```python
from build123d import *

# Parameters (mm, degrees)
SKETCH1_W               = 166
SKETCH1_H               = 196
SKETCH1_W_2             = 130
SKETCH1_H_2             = 160
BOSS_EXTRUDE1_DEPTH     = 10
CUT_EXTRUDE1_REACH      = 168
SKETCH2_R               = 2.38125
CUT_EXTRUDE2_DEPTH      = 167
SKETCH5_R               = 2.38125
CUT_EXTRUDE4_DEPTH      = 1
CUT_EXTRUDE4_DEPTH_BACK = 197
CUT_EXTRUDE5_REACH      = 12
SKETCH6_R               = 1.75
CUT_EXTRUDE7_REACH      = 22
SKETCH8_W               = 130
SKETCH8_H               = 4.5
CHAMFER9_SIZE           = 7
CHAMFER10_SIZE          = 3
CUT_EXTRUDE8_REACH      = 22
SKETCH9_R               = 1.190625
CHAMFER11_SIZE          = 3


with BuildPart() as part:
    # Sketch1 → Boss-Extrude1 (new body, symmetric)
    with BuildSketch(Plane(origin=(0, 0, 0), x_dir=(1, 0, 0), z_dir=(0, 1, 0))):
        Rectangle(SKETCH1_W, SKETCH1_H)
        Rectangle(SKETCH1_W_2, SKETCH1_H_2, mode=Mode.SUBTRACT)
    extrude(amount=BOSS_EXTRUDE1_DEPTH, both=True)

    # Sketch2 → Cut-Extrude1 (cut, up to next)
    with BuildSketch(Plane(origin=(83, 0, 0), x_dir=(0, 0, -1), z_dir=(1, 0, 0)), mode=Mode.PRIVATE) as cut_extrude1_sk1:
        Circle(SKETCH2_R)
    cut_extrude1_tool1 = extrude(cut_extrude1_sk1.sketch, amount=-CUT_EXTRUDE1_REACH, mode=Mode.PRIVATE) & part.part
    add(cut_extrude1_tool1.solids().sort_by_distance((83, 0, 0))[0], mode=Mode.SUBTRACT)

    # Sketch3 → Cut-Extrude2 (cut, through all)
    with BuildSketch(Plane.ZY.offset(83)):
        with BuildLine():
            ThreePointArc((-2.38125, 0), (0, 2.38125), (2.38125, 0))
            Line((2.38125, 0), (11, 0))
            Line((11, 0), (11, 10))
            Line((11, 10), (-11, 10))
            Line((-11, 10), (-11, 0))
            Line((-11, 0), (-2.38125, 0))
        make_face()
        with BuildLine():
            ThreePointArc((-2.38125, 0), (0, -2.38125), (2.38125, 0))
            Line((2.38125, 0), (-2.38125, 0))
        make_face()
        with BuildLine():
            Line((-2.38125, 0), (2.38125, 0))
            ThreePointArc((2.38125, 0), (0, 2.38125), (-2.38125, 0))
        make_face()
    extrude(amount=-CUT_EXTRUDE2_DEPTH, mode=Mode.SUBTRACT)

    # Sketch5 → Cut-Extrude4 (cut, two sides)
    with BuildSketch(Plane.XY.offset(98)) as cut_extrude4_sk:
        Circle(SKETCH5_R)
    extrude(amount=CUT_EXTRUDE4_DEPTH, mode=Mode.SUBTRACT)
    extrude(cut_extrude4_sk.sketch, amount=-CUT_EXTRUDE4_DEPTH_BACK, mode=Mode.SUBTRACT)

    # Sketch6 → Cut-Extrude5 (cut, up to next)
    with BuildSketch(Plane(origin=(0, 0, 0), x_dir=(1, 0, 0), z_dir=(0, 1, 0)), mode=Mode.PRIVATE) as cut_extrude5_sk1:
        with Locations((-69, 6.8)):
            Circle(SKETCH6_R)
    cut_extrude5_tool1 = extrude(cut_extrude5_sk1.sketch, amount=-CUT_EXTRUDE5_REACH, mode=Mode.PRIVATE) & part.part
    add(cut_extrude5_tool1.solids().sort_by_distance((-69, 0, -6.8))[0], mode=Mode.SUBTRACT)
    # Sketch6 → Cut-Extrude5 (cut, up to next)
    with BuildSketch(Plane(origin=(0, 0, 0), x_dir=(1, 0, 0), z_dir=(0, 1, 0)), mode=Mode.PRIVATE) as cut_extrude5_sk2:
        with Locations((-69, -6.8)):
            Circle(SKETCH6_R)
    cut_extrude5_tool2 = extrude(cut_extrude5_sk2.sketch, amount=-CUT_EXTRUDE5_REACH, mode=Mode.PRIVATE) & part.part
    add(cut_extrude5_tool2.solids().sort_by_distance((-69, 0, 6.8))[0], mode=Mode.SUBTRACT)
    # Sketch6 → Cut-Extrude5 (cut, up to next)
    with BuildSketch(Plane(origin=(0, 0, 0), x_dir=(1, 0, 0), z_dir=(0, 1, 0)), mode=Mode.PRIVATE) as cut_extrude5_sk3:
        with Locations((-79, -6.8)):
            Circle(SKETCH6_R)
    cut_extrude5_tool3 = extrude(cut_extrude5_sk3.sketch, amount=-CUT_EXTRUDE5_REACH, mode=Mode.PRIVATE) & part.part
    add(cut_extrude5_tool3.solids().sort_by_distance((-79, 0, 6.8))[0], mode=Mode.SUBTRACT)
    # Sketch6 → Cut-Extrude5 (cut, up to next)
    with BuildSketch(Plane(origin=(0, 0, 0), x_dir=(1, 0, 0), z_dir=(0, 1, 0)), mode=Mode.PRIVATE) as cut_extrude5_sk4:
        with Locations((-79, 6.8)):
            Circle(SKETCH6_R)
    cut_extrude5_tool4 = extrude(cut_extrude5_sk4.sketch, amount=-CUT_EXTRUDE5_REACH, mode=Mode.PRIVATE) & part.part
    add(cut_extrude5_tool4.solids().sort_by_distance((-79, 0, -6.8))[0], mode=Mode.SUBTRACT)
    # Sketch6 → Cut-Extrude5 (cut, up to next)
    with BuildSketch(Plane(origin=(0, 0, 0), x_dir=(1, 0, 0), z_dir=(0, 1, 0)), mode=Mode.PRIVATE) as cut_extrude5_sk5:
        with Locations((79, 6.8)):
            Circle(SKETCH6_R)
    cut_extrude5_tool5 = extrude(cut_extrude5_sk5.sketch, amount=-CUT_EXTRUDE5_REACH, mode=Mode.PRIVATE) & part.part
    add(cut_extrude5_tool5.solids().sort_by_distance((79, 0, -6.8))[0], mode=Mode.SUBTRACT)
    # Sketch6 → Cut-Extrude5 (cut, up to next)
    with BuildSketch(Plane(origin=(0, 0, 0), x_dir=(1, 0, 0), z_dir=(0, 1, 0)), mode=Mode.PRIVATE) as cut_extrude5_sk6:
        with Locations((79, -6.8)):
            Circle(SKETCH6_R)
    cut_extrude5_tool6 = extrude(cut_extrude5_sk6.sketch, amount=-CUT_EXTRUDE5_REACH, mode=Mode.PRIVATE) & part.part
    add(cut_extrude5_tool6.solids().sort_by_distance((79, 0, 6.8))[0], mode=Mode.SUBTRACT)
    # Sketch6 → Cut-Extrude5 (cut, up to next)
    with BuildSketch(Plane(origin=(0, 0, 0), x_dir=(1, 0, 0), z_dir=(0, 1, 0)), mode=Mode.PRIVATE) as cut_extrude5_sk7:
        with Locations((69, -6.8)):
            Circle(SKETCH6_R)
    cut_extrude5_tool7 = extrude(cut_extrude5_sk7.sketch, amount=-CUT_EXTRUDE5_REACH, mode=Mode.PRIVATE) & part.part
    add(cut_extrude5_tool7.solids().sort_by_distance((69, 0, 6.8))[0], mode=Mode.SUBTRACT)
    # Sketch6 → Cut-Extrude5 (cut, up to next)
    with BuildSketch(Plane(origin=(0, 0, 0), x_dir=(1, 0, 0), z_dir=(0, 1, 0)), mode=Mode.PRIVATE) as cut_extrude5_sk8:
        with Locations((69, 6.8)):
            Circle(SKETCH6_R)
    cut_extrude5_tool8 = extrude(cut_extrude5_sk8.sketch, amount=-CUT_EXTRUDE5_REACH, mode=Mode.PRIVATE) & part.part
    add(cut_extrude5_tool8.solids().sort_by_distance((69, 0, -6.8))[0], mode=Mode.SUBTRACT)

    # Sketch8 → Cut-Extrude7 (cut, up to next)
    with BuildSketch(Plane(origin=(0, 10, 0), x_dir=(1, 0, 0), z_dir=(0, 1, 0)), mode=Mode.PRIVATE) as cut_extrude7_sk1:
        with Locations((0, 82.25)):
            Rectangle(SKETCH8_W, SKETCH8_H)
    cut_extrude7_tool1 = extrude(cut_extrude7_sk1.sketch, amount=-CUT_EXTRUDE7_REACH, mode=Mode.PRIVATE) & part.part
    add(cut_extrude7_tool1.solids().sort_by_distance((0, 10, -82.25))[0], mode=Mode.SUBTRACT)
    # Sketch8 → Cut-Extrude7 (cut, up to next)
    with BuildSketch(Plane(origin=(0, 10, 0), x_dir=(1, 0, 0), z_dir=(0, 1, 0)), mode=Mode.PRIVATE) as cut_extrude7_sk2:
        with Locations((0, -82.25)):
            Rectangle(SKETCH8_W, SKETCH8_H)
    cut_extrude7_tool2 = extrude(cut_extrude7_sk2.sketch, amount=-CUT_EXTRUDE7_REACH, mode=Mode.PRIVATE) & part.part
    add(cut_extrude7_tool2.solids().sort_by_distance((0, 10, 82.25))[0], mode=Mode.SUBTRACT)

    # Chamfer9
    chamfer9_edges = [part.edges().sort_by_distance(p)[0] for p in [
        (83, 0, -98),
        (83, 0, 98),
        (-83, 0, 98),
        (-83, 0, -98),
    ]]
    chamfer(chamfer9_edges, length=CHAMFER9_SIZE)

    # Chamfer10
    chamfer10_edges = [part.edges().sort_by_distance(p)[0] for p in [
        (-65, 0, -84.5),
        (65, 0, -84.5),
        (65, 0, 84.5),
        (-65, 0, 84.5),
    ]]
    chamfer(chamfer10_edges, length=CHAMFER10_SIZE)

    # Sketch9 → Cut-Extrude8 (cut, up to next)
    with BuildSketch(Plane(origin=(0, 10, 0), x_dir=(1, 0, 0), z_dir=(0, 1, 0)), mode=Mode.PRIVATE) as cut_extrude8_sk1:
        with Locations((0, 91.25)):
            Circle(SKETCH9_R)
    cut_extrude8_tool1 = extrude(cut_extrude8_sk1.sketch, amount=-CUT_EXTRUDE8_REACH, mode=Mode.PRIVATE) & part.part
    add(cut_extrude8_tool1.solids().sort_by_distance((0, 10, -91.25))[0], mode=Mode.SUBTRACT)
    # Sketch9 → Cut-Extrude8 (cut, up to next)
    with BuildSketch(Plane(origin=(0, 10, 0), x_dir=(1, 0, 0), z_dir=(0, 1, 0)), mode=Mode.PRIVATE) as cut_extrude8_sk2:
        with Locations((0, -91.25)):
            Circle(SKETCH9_R)
    cut_extrude8_tool2 = extrude(cut_extrude8_sk2.sketch, amount=-CUT_EXTRUDE8_REACH, mode=Mode.PRIVATE) & part.part
    add(cut_extrude8_tool2.solids().sort_by_distance((0, 10, 91.25))[0], mode=Mode.SUBTRACT)

    # Chamfer11
    chamfer11_edges = [part.edges().sort_by_distance(p)[0] for p in [
        (74, 10, -11),
        (74, 10, 11),
        (-74, 10, -11),
        (-74, 10, 11),
    ]]
    chamfer(chamfer11_edges, length=CHAMFER11_SIZE)


solid = part.part
```
The listing builds one solid part. Answer for the finished solid, in the listing's coordinates (mm). A direction names the side the tool comes from. Give positions to 0.01 mm unless a question says otherwise; leave off trailing zeros. Order: outer loops, then holes, each group sorted by start corner. A loop starts at its lowest first (then second) coordinate and runs counter-clockwise, first axis right, second up. Notation, with made-up numbers: M 11,-32 L 31,-32 A7 cw 31,-23 Z; hole C -28.75,82 d7. An arc over 180 degrees is marked long. Put each result on its own line as item: value. Start each with the question number.
Item 1: For a pull along X with two mould halves and no side action, classify faces 1 (the face through (-1.1, 2.4, -98)), 2 (the face through (-79, 0, -95)), 3 (the face through (-0.9, 2.4, -84.5)) as +X half, -X half, draft (parallel to the pull), parting line (faces both ways), or undercut.
Item 2: The part is cut by section A-A, the plane z = 0. Determine the outline of the cut face in (x, y).
Item 3: Find the intervals of material crossed by line 1 along X through (y, z) = (-8, -6.8); line 2 along Z through (x, y) = (-69, -7.5); line 3 along Y through (x, z) = (0, -93), in increasing order.
Item 4: Which of the six approach directions +Z, -Z, +X, -X, +Y, -Y give full straight-line access (tool end or side, diameter ignored) to faces 4 (the face through (74, 0, -7)), 5 (the face through (-0.9, 2.4, 84.5)), 6 (the face through (-79, 0, 95))?
Item 5: The part is cut by section B-B, the plane x = -12. Determine the outline of the cut face in (y, z).
Item 6: Flat-ended cylindrical pins translate along their axes: P1, Ø3, axis at x = -69, z = 6.8, coming from the +Y side; P2, Ø4.5, axis at x = -70, z = 7.5, coming from the +Y side; P3, Ø2, axis at x = 78.5, y = 4, coming from the +Z side. Find the tip coordinate at first contact, or state that the pin passes through.
Answer key:
1. face 1: draft
1. face 2: -X half
1. face 3: undercut
2. outline: M -83,-10 L -65,-10 L -65,-2.38 L -83,-2.38 Z; M 65,-10 L 83,-10 L 83,-2.38 L 65,-2.38 Z
3. line 1: x = -83 to -80.75, -77.25 to -70.75, -67.25 to -65, 65 to 67.25, 70.75 to 77.25, 80.75 to 83
3. line 2: z = -98 to -8.55, -5.05 to 5.05, 8.55 to 98
3. line 3: y = -10 to -2.38, 2.38 to 10
4. face 4: +X, -X, +Y
4. face 5: +Y, -Y
4. face 6: +Z, -X, +Y, -Y
5. outline: M -10,-98 L 10,-98 L 10,-84.5 L -10,-84.5 Z; M -10,84.5 L 10,84.5 L 10,98 L -10,98 Z
6. P1: passes through
6. P2: stops at y = 0
6. P3: stops at z = 96.5
